For this review, take the finished solid that the model builds, in its own axes (mm). A direction names the side the tool comes from. Coordinates: 2 decimals unless noted, no trailing zeros. Loops run counter-clockwise (first coordinate to the right, second up) from the corner with the lowest first, then second, coordinate; pieces in that order, holes last. Notation, with made-up numbers: M -25,74.5 L -12,74.5 A26 ccw -12,98.5 Z; hole C 79.5,-17.5 d11. An arc over 180 degrees is marked long. Answer as a JSON object with one key per item and string values. Group by question number.
Item 1: Wall thickness on L1, parallel to Y at x = -63, z = 1.3; L2, parallel to X at y = 1.5, z = 1.35; L3, parallel to Y at x = -81.5, z = 3.75: over which ranges is each line inside the solid? List them lowest first. Write a range as from..to.
Item 2: Add section C-C (x = -50). State the section outline as (y, z) points, then the cut area to 3 significant figures.
Item 3: Tool access review of faces 4 (the face through (-94.99, 1.39, 1.97)), 5 (the face through (-78.12, 46.67, 1.97)), 6 (the face through (-41, 0, 0)): name each direction out of +Z, -Z, +X, -X, +Y, -Y from which nothing blocks a thin tool from reaching the whole face with its end or side.
Item 4: Add section D-D (y = 19). State the section outline as (x, z) points, then the cut area to 3 significant figures.
Item 5: Mouldability with a two-part tool opening along X and no side actions: class faces 1 (the face through (-77.455, -47.767, 1.972)), 2 (the face through (-45.726, 89.197, 1.972)), 3 (the face through (-41, 0, 4)) as +X half, -X half, draft (parallel to the pull), parting line (faces both ways), or undercut.
Item 6: Add section B-B (z = 0.7). State the section outline as (x, y) points.
Item 7: Add section A-A (y = -66). State the section outline as (x, z) points, then the cut area to 3 significant figures.
Item 8: Insertion check: pin 1 (2 mm diameter, centred on y = 43.5, z = 3.5, fed in from -X); pin 2 (2 mm diameter, centred on x = 36.5, z = 3, fed in from +Y); pin 3 (2 mm diameter, centred on y = -49, z = 3, fed in from -X). Each pin has a flat end and moves straight along its axis. Give the tip position at first contact, or say it passes through.
from build123d import *

# Parameters (mm, degrees)
EXTRUDE_1_DEPTH = 4


with BuildPart() as part:
    # 草图1 → 凸台-拉伸1 (new body)
    with BuildSketch(Plane.XY):
        with BuildLine():
            Line((-90.912045407, -4), (0, -4))
            Line((0, -4), (109, -4))
            Line((109, -4), (109, 4))
            Line((109, 4), (0, 4))
            Line((0, 4), (-90.912045407, 4))
            ThreePointArc((-90.912045407, 4), (-77.789024994, 47.221473828), (-45.5, 78.808311744))
            ThreePointArc((-45.5, 78.808311744), (-42.205771366, 91.102540378), (-54.5, 94.396769013))
            ThreePointArc((-54.5, 94.396769013), (-109, 0), (-54.5, -94.396769013))
            ThreePointArc((-54.5, -94.396769013), (-42.205771366, -91.102540378), (-45.5, -78.808311744))
            ThreePointArc((-45.5, -78.808311744), (-77.789024994, -47.221473828), (-90.912045407, -4))
        make_face()
        with BuildLine():
            ThreePointArc((-52.5, -90.932667397), (-105, 0), (-52.5, 90.932667397))
            ThreePointArc((-52.5, 90.932667397), (-45.669872981, 89.102540378), (-47.5, 82.27241336))
            ThreePointArc((-47.5, 82.27241336), (-95, 0), (-47.5, -82.27241336))
            ThreePointArc((-47.5, -82.27241336), (-45.669872981, -89.102540378), (-52.5, -90.932667397))
        make_face(mode=Mode.SUBTRACT)
    extrude(amount=EXTRUDE_1_DEPTH)


solid = part.part
From the geometry:
{
 "1": {"L1": "y = -88.95..-84, -71.11..-65.67, -4..4, 65.67..71.11, 84..88.95", "L2": "x = -108.99..-104.99, -94.99..109", "L3": "y = -72.38..-66.2, -48.81..-40.48, -4..4, 40.48..48.81, 66.2..72.38"},
 "2": {"outline": "M -95.6,0 L -91.6,0 L -91.6,4 L -95.6,4 Z; M -80.78,0 L -76.03,0 L -76.03,4 L -80.78,4 Z; M -4,0 L 4,0 L 4,4 L -4,4 Z; M 76.03,0 L 80.78,0 L 80.78,4 L 76.03,4 Z; M 91.6,0 L 95.6,0 L 95.6,4 L 91.6,4 Z", "area": "102 mm²"},
 "3": {"face 4": "+Z, -Z", "face 5": "+Z, -Z, +X", "face 6": "-Z, +X, -X, +Y, -Y"},
 "4": {"outline": "M -107.33,0 L -103.27,0 L -103.27,4 L -107.33,4 Z; M -93.08,0 L -88.99,0 L -88.99,4 L -93.08,4 Z", "area": "32.6 mm²"},
 "5": {"face 1": "+X half", "face 2": "undercut", "face 3": "draft"},
 "6": {"outline": "M -90.91,-4 L 109,-4 L 109,4 L -90.91,4 A91 cw -45.5,78.81 A9 ccw -54.5,94.4 A109 ccw -54.5,-94.4 A9 ccw -45.5,-78.81 A91 cw Z; hole M -52.5,-90.93 A5 ccw -47.5,-82.27 A95 cw -47.5,82.27 A5 ccw -52.5,90.93 A105 ccw Z"},
 "7": {"outline": "M -86.75,0 L -81.66,0 L -81.66,4 L -86.75,4 Z; M -68.33,0 L -62.65,0 L -62.65,4 L -68.33,4 Z", "area": "43.1 mm²"},
 "8": {"pin 1": "stops at x = -100.37", "pin 2": "stops at y = 4", "pin 3": "stops at x = -97.86"}
}
